from build123d import *

# Parameters (mm, degrees)
SKETCH_W          = 37
SKETCH_H          = 34
PAD_DEPTH         = 4.5
FILLET_R          = 2
SKETCH001_W       = 26
SKETCH001_H       = 25
PAD001_DEPTH      = 5.5
FILLET001_R       = 3
SKETCH002_R       = 2.55
POCKET_DEPTH      = 4.501
POCKET_DEPTH_BACK = -5.501


with BuildPart() as part:
    # Sketch → Pad (new body)
    with BuildSketch(Plane.XZ):
        with Locations((0, 7)):
            Rectangle(SKETCH_W, SKETCH_H)
    extrude(amount=-PAD_DEPTH)

    # Fillet
    fillet_edges = [part.edges().sort_by_distance(p)[0] for p in [
        (18.5, 2.25, 24),
        (-18.5, 2.25, 24),
        (18.5, 2.25, -10),
        (-18.5, 2.25, -10),
    ]]
    fillet(fillet_edges, radius=FILLET_R)

    # Sketch001 → Pad001 (join)
    with BuildSketch(Plane.XZ):
        with Locations((0, 5.5)):
            Rectangle(SKETCH001_W, SKETCH001_H)
    extrude(amount=PAD001_DEPTH)

    # Fillet001
    fillet001_edges = [part.edges().sort_by_distance(p)[0] for p in [
        (-13, -2.75, -7),
        (13, -2.75, -7),
        (-13, -2.75, 18),
        (13, -2.75, 18),
    ]]
    fillet(fillet001_edges, radius=FILLET001_R)

    # Sketch002 → Pocket (cut, two sides)
    with BuildSketch(Plane.XZ) as pocket_sk:
        Circle(SKETCH002_R)
    extrude(amount=-POCKET_DEPTH, mode=Mode.SUBTRACT)
    extrude(pocket_sk.sketch, amount=-POCKET_DEPTH_BACK, mode=Mode.SUBTRACT)


solid = part.part
The listing builds one solid part. Answer for the finished solid, in the listing's coordinates (mm). A direction names the side the tool comes from. Coordinates: 2 decimals unless noted, no trailing zeros. Order: outer loops, then holes, each group sorted by start corner. A loop starts at its lowest first (then second) coordinate and runs counter-clockwise, first axis right, second up. Notation, with made-up numbers: M -35,-33.5 L 22,-33.5 A19 cw 22,-15.5 Z; hole C 69,20.25 d10. An arc over 180 degrees is marked long. Use CSV: the item, a comma, the result in double quotes.
Q1. Section C-C (z = 0) is taken. Determine the outline of the cut face in (x, y), then the cut area to 4 significant figures.
Here are the results:
outline,"M -18.5,0 L -13,0 L -13,-5.5 L -2.55,-5.5 L -2.55,4.5 L -18.5,4.5 Z; M 2.55,-5.5 L 13,-5.5 L 13,0 L 18.5,0 L 18.5,4.5 L 2.55,4.5 Z"
area,"258.5 mm2"
Q2. A tool of negligible diameter and unlimited length cuts with its end or side. For faces 1 (the flat face through (-13, -3, 5)), 2 (the flat face through (0, -3, 18)), 3 (the flat face through (0, -3, -7)), 4 (the cylindrical face through (12.1, -2.79, -6.14)), from which of +Z, -Z, +X, -X, +Y, -Y can it reach the whole face along a straight path? Write none if from no direction.
Here are the results:
face 1,"+Z, -Z, -X, -Y"
face 2,"+Z, +X, -X, -Y"
face 3,"-Z, +X, -X, -Y"
face 4,"-Z, +X, -Y"
Q3. Given pin 1 Ø1.6 at (y, z) = (-2, 10) entering from +X; pin 2 Ø4.5 at (x, z) = (0, 0) entering from +Y; pin 3 Ø1.6 at (x, y) = (2, -3) entering from -Z; pin 4 Ø4 at (x, y) = (13, -2.5) entering from -Z, each flat-ended and moving along its own axis, determine where each tip first touches the part or whether it passes through.
Here are the results:
pin 1,"x = 13"
pin 2,"through"
pin 3,"z = -7"
pin 4,"z = -6.83"
Q4. Section D-D (z = 10) is taken. Determine the outline of the cut face in (x, y), then the cut area to 4 significant figures.
Here are the results:
outline,"M -18.5,0 L -13,0 L -13,-5.5 L 13,-5.5 L 13,0 L 18.5,0 L 18.5,4.5 L -18.5,4.5 Z"
area,"309.5 mm2"
Q5. Section A-A (x = 0) is taken. Determine the outline of the cut face in (y, z).
Here are the results:
outline,"M -5.5,-7 L 0,-7 L 0,-10 L 4.5,-10 L 4.5,-2.55 L -5.5,-2.55 Z; M -5.5,2.55 L 4.5,2.55 L 4.5,24 L 0,24 L 0,18 L -5.5,18 Z"
Q6. Straight lines are drawn through the part: L1, parallel to Z at x = 0, y = -3.2; L2, parallel to X at y = -3.5, z = 0; L3, parallel to Y at x = -13, z = 16.5. For each, find the intervals that lie inside material, in ascending order.
Here are the results:
L1,"-7 to -2.55, 2.55 to 18"
L2,"-13 to -2.55, 2.55 to 13"
L3,"0 to 4.5"
Q7. Section B-B (y = -1) is taken. Determine the outline of the cut face in (x, z), then the cut area to 3 significant figures.
Here are the results:
outline,"M -13,-4 A3 ccw -10,-7 L 10,-7 A3 ccw 13,-4 L 13,15 A3 ccw 10,18 L -10,18 A3 ccw -13,15 Z; hole C 0,0 d5.1"
area,"622 mm2"
